Could you check a few things on this model? Use its own coordinates, in mm. Face numbers are marked on the shaded views. A direction names the side the tool comes from. Give positions to 0.01 mm unless a question says otherwise; leave off trailing zeros. Order: outer loops, then holes, each group sorted by start corner. A loop starts at its lowest first (then second) coordinate and runs counter-clockwise, first axis right, second up. Notation, with made-up numbers: (43.25, -22.75) - (54.25, -22.75) arc R29 ccw to (54.25, -2.75) - close; hole circle Ø8 at (13.25, 10.5). An arc over 180 degrees is marked (long way). Put each result on its own line as item: value.
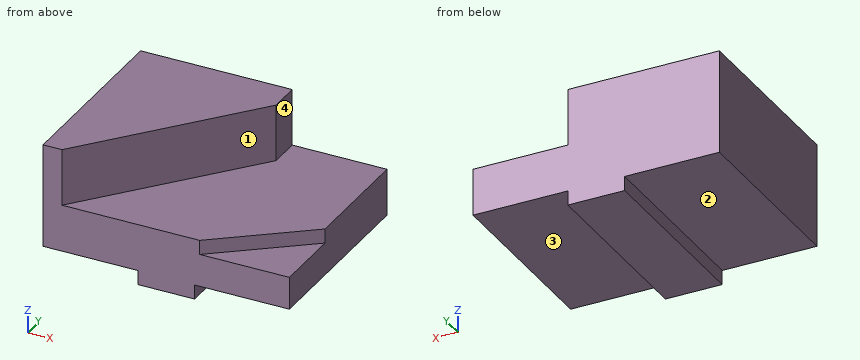
from build123d import *

# Parameters (mm, degrees)
F0_W     = 82.55
F0_H     = 39.624
F1_DEPTH = 63.5
F2_W     = 31.75
F2_H     = 4.826
F3_DEPTH = 153.924
F4_W     = 31.75
F4_H     = 4.826
F5_DEPTH = 83.058
F7_DEPTH = 19.05
F9_DEPTH = 4.826


with BuildPart() as f1:
    # F0 (on Front) → F1 (new body)
    with BuildSketch(Plane.XZ):
        with Locations((-5.060298, -1.674932)):
            Rectangle(F0_W, F0_H)
    extrude(amount=-F1_DEPTH)

    # F2 (on face) → F3 (cut)
    with BuildSketch(Plane.XZ):
        with Locations((-30.460298, -19.073932)):
            Rectangle(F2_W, F2_H)
    extrude(amount=-F3_DEPTH, mode=Mode.SUBTRACT)

    # F4 (on face) → F5 (cut)
    with BuildSketch(Plane.XZ):
        with Locations((20.339702, -19.073932)):
            Rectangle(F4_W, F4_H)
    extrude(amount=-F5_DEPTH, mode=Mode.SUBTRACT)

    # F6 (on face) → F7 (cut)
    with BuildSketch(Plane.XY.offset(18.137068)):
        Polygon((36.214702, 63.5), (4.464702, 63.5), (4.464702, 52.973447), (-39.985298, 0), (36.214702, 0), align=None)
    extrude(amount=-F7_DEPTH, mode=Mode.SUBTRACT)

    # F8 (on face) → F9 (cut)
    with BuildSketch(Plane.XY.offset(-0.912932)):
        Polygon((36.214702, 23.16233), (6.150608, 0), (36.214702, 0), align=None)
    extrude(amount=-F9_DEPTH, mode=Mode.SUBTRACT)


solid = f1.part
1) If I drill on line 1 (Z direction, x = -38, y = 30); line 2 (Z direction, x = -19, y = 5); line 3 (X direction, y = 53, z = 5), over which ranges is the centre line in solid material (lowest first)? Write a range as [from, to].
Filled in:
line 1: z = [-16.66, 18.14]
line 2: z = [-16.66, -0.91]
line 3: x = [-46.34, 4.46]
2) Which directions (+Z, -Z, +X, -X, +Y, -Y) give clear straight access to the entire face, cutting with the end or side of a thin tool? Please do the marked faces 1, 2, 3 and 4.
Filled in:
face 1: +Z, +X, -Y
face 2: -Z, -X, +Y, -Y
face 3: -Z, +X, +Y, -Y
face 4: +Z, +X, +Y, -Y
3) Suppose I cut it at C-C, the plane x = -36. List the corners of the cut face in (y, z) for me, and give its area (3 significant figures).
Filled in:
outline: (0, -16.66) - (63.5, -16.66) - (63.5, 18.14) - (4.75, 18.14) - (4.75, -0.91) - (0, -0.91) - close
area: 2,120 mm^2
4) Suppose I cut it at D-D, the plane y = 15. List the corners of the cut face in (x, z) for me.
Filled in:
outline: (-46.34, -16.66) - (-14.59, -16.66) - (-14.59, -21.49) - (4.46, -21.49) - (4.46, -16.66) - (36.21, -16.66) - (36.21, -5.74) - (25.62, -5.74) - (25.62, -0.91) - (-27.4, -0.91) - (-27.4, 18.14) - (-46.34, 18.14) - close
5) Suppose I cut it at B-B, the plane y = 25.5. List the corners of the cut face in (x, z) for me, and give its area (3 significant figures).
Filled in:
outline: (-46.34, -16.66) - (-14.59, -16.66) - (-14.59, -21.49) - (4.46, -21.49) - (4.46, -16.66) - (36.21, -16.66) - (36.21, -0.91) - (-18.59, -0.91) - (-18.59, 18.14) - (-46.34, 18.14) - close
area: 1,920 mm^2
6) I'm going to push flat-ended pins straight in: pin 1 (18.5 mm diameter, centred on x = 22.5, y = 15, fed in from +Z); pin 2 (3 mm diameter, centred on y = 56, z = 10.5, fed in from +X); pin 3 (9.5 mm diameter, centred on x = -31, y = 36.5, fed in from -Z). Where does each tip first touch, or does it pass through?
Filled in:
pin 1: stops at z = -0.91
pin 2: stops at x = 4.46
pin 3: stops at z = -16.66
7) Suppose I cut it at A-A, the plane z = 6.5. List the corners of the cut face in (x, y) for me, and give its area (3 significant figures).
Filled in:
outline: (-46.34, 0) - (-39.99, 0) - (4.46, 52.97) - (4.46, 63.5) - (-46.34, 63.5) - close
area: 2,050 mm^2
